Geometry check sheet. Reference: drawing and pictorial views, mm from the part's lowest x, y, z. A direction names the side the tool comes from. Coordinates: 2 decimals unless noted, no trailing zeros. Loops run counter-clockwise (first coordinate to the right, second up) from the corner with the lowest first, then second, coordinate; pieces in that order, holes last.
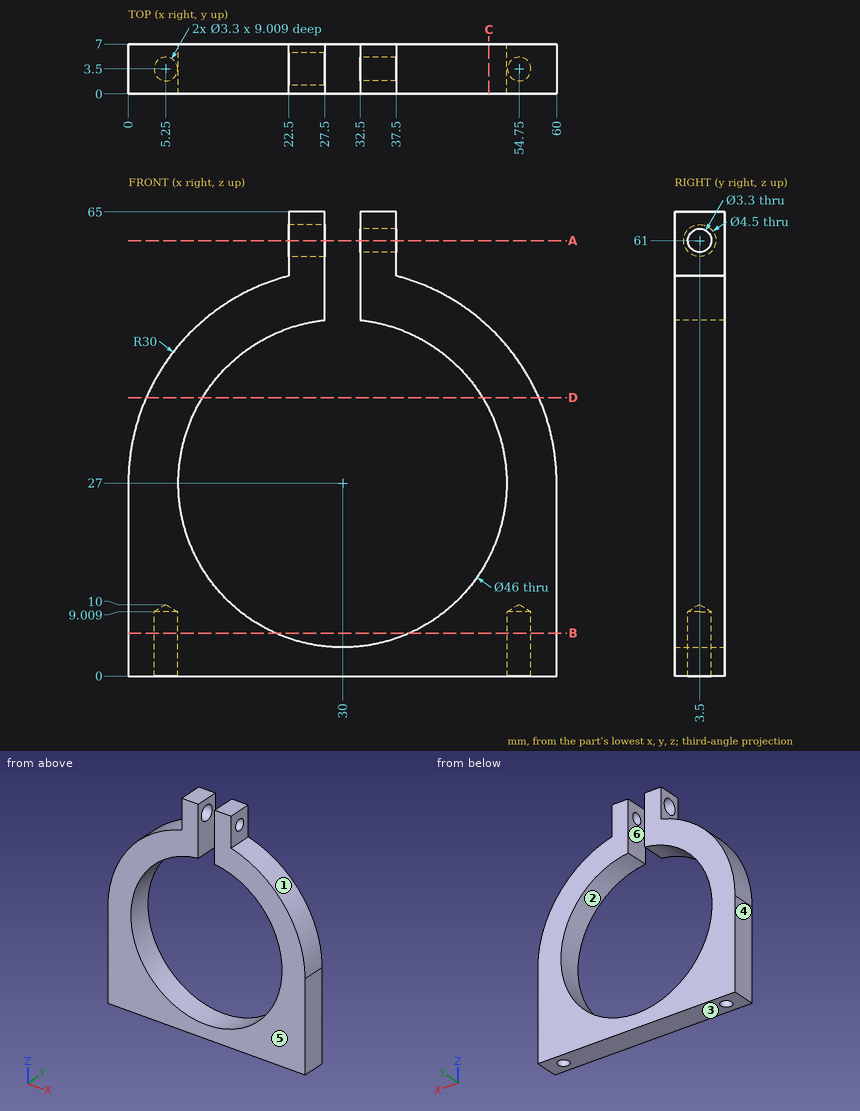
1) Section check B-B on z = 6. Record the cut outline in (x, y).
Data:
outline: (0, 0) - (20.62, 0) - (20.62, 7) - (0, 7) - close; (39.38, 0) - (60, 0) - (60, 7) - (39.38, 7) - close; hole circle Ø3.3 at (5.25, 3.5); hole circle Ø3.3 at (54.75, 3.5)
2) Depth check by flat-ended pin: pin 1 (3.5 mm diameter, centred on y = 3.5, z = 61, fed in from +X); pin 2 (4 mm diameter, centred on x = 6.5, y = 5, fed in from -Z); pin 3 (1.5 mm diameter, centred on x = 12, y = 2, fed in from +Z) (1 decimal); pin 4 (2 mm diameter, centred on y = 5.5, z = 41.5, fed in from +X). Enter the tip coordinate at first touch or a pass-through.
Data:
pin 1: stops at x = 37.5
pin 2: stops at z = 0
pin 3: stops at z = 51.5
pin 4: stops at x = 56.79
3) Material ranges on probe 1 along X at (y, z) = (3.5, 3.5); probe 2 along Y at (x, z) = (54.75, 2.75); probe 3 along X at (y, z) = (3.5, 27), recorded low to high.
Data:
probe 1: x = 0 to 3.6, 6.9 to 53.1, 56.4 to 60
probe 2: y = 0 to 1.85, 5.15 to 7
probe 3: x = 0 to 7, 53 to 60
4) Section check C-C on x = 50.5. Record the cut outline in (y, z), and give its area (3 significant figures).
Data:
outline: (0, 0) - (7, 0) - (7, 16.57) - (0, 16.57) - close; (0, 37.43) - (7, 37.43) - (7, 48.9) - (0, 48.9) - close
area: 196 mm2
5) Section check D-D on z = 39. Record the cut outline in (x, y) (1 decimal), and give its area (3 significant figures).
Data:
outline: (2.5, 0) - (10.4, 0) - (10.4, 7) - (2.5, 7) - close; (49.6, 0) - (57.5, 0) - (57.5, 7) - (49.6, 7) - close
area: 110 mm2
6) Section check A-A on z = 61. Record the cut outline in (x, y), and give its area (3 significant figures).
Data:
outline: (22.5, 0) - (27.5, 0) - (27.5, 1.25) - (22.5, 1.25) - close; (22.5, 5.75) - (27.5, 5.75) - (27.5, 7) - (22.5, 7) - close; (32.5, 0) - (37.5, 0) - (37.5, 1.85) - (32.5, 1.85) - close; (32.5, 5.15) - (37.5, 5.15) - (37.5, 7) - (32.5, 7) - close
area: 31.0 mm2
7) Access from +Z, -Z, +X, -X, +Y, -Y to the whole of each face (thin tool, end or side, straight path). Record for the marked faces 5 and 6.
Data:
face 5: +Z, -Z, +X, -X, -Y
face 6: +Z, +Y, -Y
8) Mould release check, pull along Z, two halves, no side actions. Record for the marked faces 1, 2, 3 and 4: +Z half, -Z half, draft (parallel to the pull), parting line (faces both ways), or undercut.
Data:
face 1: +Z half
face 2: undercut
face 3: -Z half
face 4: draft
